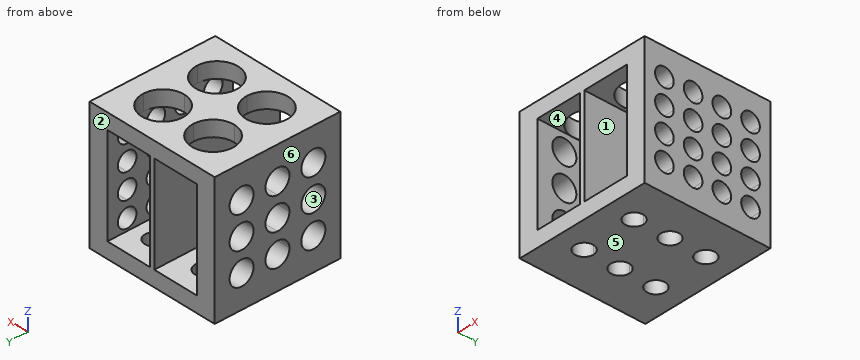
from build123d import *

# Parameters (mm, degrees)
F0_W          = 95.25
F0_H          = 88.9
F1_DEPTH      = 46.0375
F1_DEPTH_BACK = 46.0375
F2_W          = 32.54375
F2_H          = 69.85
F3_DEPTH      = 88.9
F5_DEPTH      = 11.1125
F6_R          = 8.509
F7_DEPTH      = 13.49375
F8_R          = 6.604
F9_DEPTH      = 11.1125
F11_DEPTH     = 13.49375


with BuildPart() as f1:
    # F0 (on Top) → F1 (new body, two sides)
    with BuildSketch(Plane.XY) as f1_sk:
        Rectangle(F0_W, F0_H)
    extrude(amount=F1_DEPTH)
    extrude(f1_sk.sketch, amount=-F1_DEPTH_BACK)

    # F2 (on face) → F3 (cut, through all)
    with BuildSketch(Plane.XZ.offset(44.45)):
        with Locations((17.859375, 0)):
            Rectangle(F2_W, F2_H)
        with Locations((-17.859375, 0)):
            Rectangle(F2_W, F2_H)
    extrude(amount=-F3_DEPTH, mode=Mode.SUBTRACT)

    # F4 (on face) → F5 (cut, through all)
    with BuildSketch(Plane.XY.offset(46.0375)):
        with BuildLine():
            ThreePointArc((-4.05003, 19.05), (-29.6565805046, 29.6565805046), (-19.05, 4.05003))
            ThreePointArc((-19.05, 4.05003), (-8.4434194954, 8.4434194954), (-4.05003, 19.05))
        make_face()
        with BuildLine():
            ThreePointArc((34.04997, 19.05), (8.4434194954, 29.6565805046), (19.05, 4.05003))
            ThreePointArc((19.05, 4.05003), (29.6565805046, 8.4434194954), (34.04997, 19.05))
        make_face()
        with BuildLine():
            ThreePointArc((34.04997, -19.05), (29.6565805046, -8.4434194954), (19.05, -4.05003))
            ThreePointArc((19.05, -4.05003), (8.4434194954, -29.6565805046), (34.04997, -19.05))
        make_face()
        with BuildLine():
            ThreePointArc((-4.05003, -19.05), (-8.4434194954, -8.4434194954), (-19.05, -4.05003))
            ThreePointArc((-19.05, -4.05003), (-29.6565805046, -29.6565805046), (-4.05003, -19.05))
        make_face()
    extrude(amount=-F5_DEPTH, mode=Mode.SUBTRACT)

    # F6 (on face) → F7 (cut, through all)
    with BuildSketch(Plane(origin=(-47.625, 0, 0), x_dir=(0, -1, 0), z_dir=(-1, 0, 0))):
        with BuildLine():
            ThreePointArc((0, -8.509), (6.0167716011, -6.0167716011), (8.509, 0))
            ThreePointArc((8.509, 0), (6.0167716011, 6.0167716011), (0, 8.509))
            Line((0, 8.509), (0, 0))
            Line((0, 0), (0, -8.509))
        make_face()
        with BuildLine():
            ThreePointArc((8.509, -22.86), (6.0167716011, -16.8432283989), (0, -14.351))
            ThreePointArc((0, -14.351), (-6.0167716011, -28.8767716011), (8.509, -22.86))
        make_face()
        with BuildLine():
            ThreePointArc((8.509, 22.86), (-6.0167716011, 28.8767716011), (0, 14.351))
            ThreePointArc((0, 14.351), (6.0167716011, 16.8432283989), (8.509, 22.86))
        make_face()
        with BuildLine():
            Line((0, 0), (0, 8.509))
            ThreePointArc((0, 8.509), (-8.509, 0), (0, -8.509))
            Line((0, -8.509), (0, 0))
        make_face()
        with Locations((-25.4, 22.86)):
            Circle(F6_R)
        with Locations((-25.4, 0)):
            Circle(F6_R)
        with Locations((-25.4, -22.86)):
            Circle(F6_R)
        with Locations((25.4, 22.86)):
            Circle(F6_R)
        with Locations((25.4, 0)):
            Circle(F6_R)
        with Locations((25.4, -22.86)):
            Circle(F6_R)
    extrude(amount=-F7_DEPTH, mode=Mode.SUBTRACT)

    # F8 (on face) → F9 (cut, through all)
    with BuildSketch(Plane(origin=(0, 0, -46.0375), x_dir=(1, 0, 0), z_dir=(0, 0, -1))):
        with BuildLine():
            ThreePointArc((-19.05, -6.604), (-14.380266817, -4.669733183), (-12.446, 0))
            Line((-12.446, 0), (-19.05, 0))
            Line((-19.05, 0), (-19.05, -6.604))
        make_face()
        with BuildLine():
            Line((-19.05, 0), (-12.446, 0))
            ThreePointArc((-12.446, 0), (-14.380266817, 4.669733183), (-19.05, 6.604))
            Line((-19.05, 6.604), (-19.05, 0))
        make_face()
        with BuildLine():
            ThreePointArc((-12.446, -25.4), (-14.380266817, -20.730266817), (-19.05, -18.796))
            ThreePointArc((-19.05, -18.796), (-23.719733183, -30.069733183), (-12.446, -25.4))
        make_face()
        with BuildLine():
            ThreePointArc((-12.446, 25.4), (-23.719733183, 30.069733183), (-19.05, 18.796))
            ThreePointArc((-19.05, 18.796), (-14.380266817, 20.730266817), (-12.446, 25.4))
        make_face()
        with BuildLine():
            Line((-19.05, -6.604), (-19.05, 0))
            Line((-19.05, 0), (-19.05, 6.604))
            ThreePointArc((-19.05, 6.604), (-25.654, 0), (-19.05, -6.604))
        make_face()
        with BuildLine():
            ThreePointArc((19.05, 18.796), (23.719733183, 20.730266817), (25.654, 25.4))
            ThreePointArc((25.654, 25.4), (14.380266817, 30.069733183), (19.05, 18.796))
        make_face()
        with BuildLine():
            ThreePointArc((25.654, 0), (23.719733183, 4.669733183), (19.05, 6.604))
            ThreePointArc((19.05, 6.604), (14.380266817, -4.669733183), (25.654, 0))
        make_face()
        with Locations((19.05, -25.4)):
            Circle(F8_R)
    extrude(amount=-F9_DEPTH, mode=Mode.SUBTRACT)

    # F10 (on face) → F11 (cut, through all)
    with BuildSketch(Plane.YZ.offset(47.625)):
        with BuildLine():
            ThreePointArc((-23.876, -26.67), (-25.810266817, -22.000266817), (-30.48, -20.066))
            ThreePointArc((-30.48, -20.066), (-35.149733183, -31.339733183), (-23.876, -26.67))
        make_face()
        with BuildLine():
            ThreePointArc((-23.876, -8.89), (-25.810266817, -4.220266817), (-30.48, -2.286))
            Line((-30.48, -2.286), (-30.48, -8.89))
            Line((-30.48, -8.89), (-30.48, -15.494))
            ThreePointArc((-30.48, -15.494), (-25.810266817, -13.559733183), (-23.876, -8.89))
        make_face()
        with BuildLine():
            Line((-30.48, -8.89), (-30.48, -2.286))
            ThreePointArc((-30.48, -2.286), (-37.084, -8.89), (-30.48, -15.494))
            Line((-30.48, -15.494), (-30.48, -8.89))
        make_face()
        with BuildLine():
            ThreePointArc((-23.876, 26.67), (-35.149733183, 31.339733183), (-30.48, 20.066))
            ThreePointArc((-30.48, 20.066), (-25.810266817, 22.000266817), (-23.876, 26.67))
        make_face()
        with BuildLine():
            ThreePointArc((-30.48, 15.494), (-37.084, 8.89), (-30.48, 2.286))
            Line((-30.48, 2.286), (-30.48, 8.89))
            Line((-30.48, 8.89), (-30.48, 15.494))
        make_face()
        with BuildLine():
            Line((-30.48, 8.89), (-30.48, 2.286))
            ThreePointArc((-30.48, 2.286), (-25.810266817, 4.220266817), (-23.876, 8.89))
            ThreePointArc((-23.876, 8.89), (-25.810266817, 13.559733183), (-30.48, 15.494))
            Line((-30.48, 15.494), (-30.48, 8.89))
        make_face()
        with BuildLine():
            ThreePointArc((-3.556, -26.67), (-5.490266817, -22.000266817), (-10.16, -20.066))
            ThreePointArc((-10.16, -20.066), (-14.829733183, -31.339733183), (-3.556, -26.67))
        make_face()
        with BuildLine():
            ThreePointArc((-3.556, -8.89), (-5.490266817, -4.220266817), (-10.16, -2.286))
            Line((-10.16, -2.286), (-10.16, -8.89))
            Line((-10.16, -8.89), (-10.16, -15.494))
            ThreePointArc((-10.16, -15.494), (-5.490266817, -13.559733183), (-3.556, -8.89))
        make_face()
        with BuildLine():
            Line((-10.16, -8.89), (-10.16, -2.286))
            ThreePointArc((-10.16, -2.286), (-16.764, -8.89), (-10.16, -15.494))
            Line((-10.16, -15.494), (-10.16, -8.89))
        make_face()
        with BuildLine():
            ThreePointArc((-3.556, 26.67), (-14.829733183, 31.339733183), (-10.16, 20.066))
            ThreePointArc((-10.16, 20.066), (-5.490266817, 22.000266817), (-3.556, 26.67))
        make_face()
        with BuildLine():
            ThreePointArc((-10.16, 15.494), (-16.764, 8.89), (-10.16, 2.286))
            Line((-10.16, 2.286), (-10.16, 8.89))
            Line((-10.16, 8.89), (-10.16, 15.494))
        make_face()
        with BuildLine():
            Line((-10.16, 8.89), (-10.16, 2.286))
            ThreePointArc((-10.16, 2.286), (-5.490266817, 4.220266817), (-3.556, 8.89))
            ThreePointArc((-3.556, 8.89), (-5.490266817, 13.559733183), (-10.16, 15.494))
            Line((-10.16, 15.494), (-10.16, 8.89))
        make_face()
        with BuildLine():
            ThreePointArc((10.16, 20.066), (14.829733183, 22.000266817), (16.764, 26.67))
            ThreePointArc((16.764, 26.67), (5.490266817, 31.339733183), (10.16, 20.066))
        make_face()
        with BuildLine():
            ThreePointArc((16.764, -26.67), (14.829733183, -22.000266817), (10.16, -20.066))
            ThreePointArc((10.16, -20.066), (5.490266817, -31.339733183), (16.764, -26.67))
        make_face()
        with BuildLine():
            ThreePointArc((16.764, -8.89), (14.829733183, -4.220266817), (10.16, -2.286))
            Line((10.16, -2.286), (10.16, -8.89))
            Line((10.16, -8.89), (10.16, -15.494))
            ThreePointArc((10.16, -15.494), (14.829733183, -13.559733183), (16.764, -8.89))
        make_face()
        with BuildLine():
            Line((10.16, -8.89), (10.16, -2.286))
            ThreePointArc((10.16, -2.286), (3.556, -8.89), (10.16, -15.494))
            Line((10.16, -15.494), (10.16, -8.89))
        make_face()
        with BuildLine():
            ThreePointArc((16.764, 8.89), (14.829733183, 13.559733183), (10.16, 15.494))
            Line((10.16, 15.494), (10.16, 8.89))
            Line((10.16, 8.89), (10.16, 2.286))
            ThreePointArc((10.16, 2.286), (14.829733183, 4.220266817), (16.764, 8.89))
        make_face()
        with BuildLine():
            Line((10.16, 8.89), (10.16, 15.494))
            ThreePointArc((10.16, 15.494), (3.556, 8.89), (10.16, 2.286))
            Line((10.16, 2.286), (10.16, 8.89))
        make_face()
        with BuildLine():
            ThreePointArc((30.48, 20.066), (35.149733183, 22.000266817), (37.084, 26.67))
            ThreePointArc((37.084, 26.67), (25.810266817, 31.339733183), (30.48, 20.066))
        make_face()
        with BuildLine():
            ThreePointArc((37.084, -26.67), (35.149733183, -22.000266817), (30.48, -20.066))
            ThreePointArc((30.48, -20.066), (25.810266817, -31.339733183), (37.084, -26.67))
        make_face()
        with BuildLine():
            ThreePointArc((37.084, -8.89), (35.149733183, -4.220266817), (30.48, -2.286))
            Line((30.48, -2.286), (30.48, -8.89))
            Line((30.48, -8.89), (30.48, -15.494))
            ThreePointArc((30.48, -15.494), (35.149733183, -13.559733183), (37.084, -8.89))
        make_face()
        with BuildLine():
            Line((30.48, -8.89), (30.48, -2.286))
            ThreePointArc((30.48, -2.286), (23.876, -8.89), (30.48, -15.494))
            Line((30.48, -15.494), (30.48, -8.89))
        make_face()
        with BuildLine():
            ThreePointArc((37.084, 8.89), (35.149733183, 13.559733183), (30.48, 15.494))
            Line((30.48, 15.494), (30.48, 8.89))
            Line((30.48, 8.89), (30.48, 2.286))
            ThreePointArc((30.48, 2.286), (35.149733183, 4.220266817), (37.084, 8.89))
        make_face()
        with BuildLine():
            Line((30.48, 8.89), (30.48, 15.494))
            ThreePointArc((30.48, 15.494), (23.876, 8.89), (30.48, 2.286))
            Line((30.48, 2.286), (30.48, 8.89))
        make_face()
    extrude(amount=-F11_DEPTH, mode=Mode.SUBTRACT)


solid = f1.part
Work out the finished part from the listing and answer in its coordinate system (mm). Face numbers are marked on the shaded views. A direction names the side the tool comes from. Give positions to 0.01 mm unless a question says otherwise; leave off trailing zeros. Use a Markdown table: item, result. Add a question column.
1. Find the intervals of material crossed by probe 1 along X at (y, z) = (10, 33.5) (1 decimal); probe 2 along Y at (x, z) = (41.5, -26.67); probe 3 along X at (y, z) = (-25, -40) (3 decimals), in increasing order.
2. Flat-ended cylindrical pins translate along their axes: pin 1 Ø16.5 at (x, y) = (23, -14) entering from +Z (3 decimals); pin 2 Ø10.5 at (y, z) = (-10.16, -26.67) entering from +X. Find the tip coordinate at first contact, or state that the pin passes through.
3. For the marked faces 1, 2 and 3, determine the directions among +Z, -Z, +X, -X, +Y, -Y from which every point of the face is accessible in a straight line to the end or side of a thin tool.
4. Section A-A on x = -38.5 is taken. State how many separate pieces and enclosed holes the cut face has, and give its area (3 significant figures).
5. Determine the mould class of the marked faces 4, 5 and 6 for opening direction Z: released by +Z, released by -Z, zero draft, split by the parting line, or undercut.
Results below:
| question | item | result |
|---|---|---|
| 1 | probe 1 | x = -47.6 to -34.1, -1.6 to 1.6, 34.1 to 47.6 |
| 1 | probe 2 | y = -44.45 to -37.08, -23.88 to -16.76, -3.56 to 3.56, 16.76 to 23.88, 37.08 to 44.45 |
| 1 | probe 3 | x = -47.625 to -25.642, -12.458 to 12.458, 25.642 to 47.625 |
| 2 | pin 1 | stops at z = -34.925 |
| 2 | pin 2 | stops at x = 1.59 |
| 3 | face 1 | +Y, -Y |
| 3 | face 2 | +Z, -Z, +X, -X, +Y |
| 3 | face 3 | -X |
| 4 | separate pieces | 1 |
| 4 | enclosed holes | 9 |
| 4 | area | 6,140 mm^2 |
| 5 | face 4 | undercut |
| 5 | face 5 | released by -Z |
| 5 | face 6 | zero draft |
